Here's how the part is built. I have some questions about the finished solid (model axes, mm). A direction names the side the tool comes from. Round coordinates to 2 decimals unless told otherwise and drop trailing zeros. Loops run counter-clockwise (first coordinate to the right, second up) from the corner with the lowest first, then second, coordinate; pieces in that order, holes last. Notation, with made-up numbers: M 31.25,-23 L 44.25,-23 A12 cw 44.25,-9 Z; hole C 43.25,-3 d1. An arc over 180 degrees is marked long. Answer as CSV lines item,"result".
```python
from build123d import *


with BuildPart() as part:
    # Sweep1: sweep along a path in Sketch2
    with BuildLine(Plane.XY) as sweep1_path:
        Line((0.760799283, -6.022132882), (48.345774261, -0.010539388))
        ThreePointArc((48.345774261, -0.010539388), (62.299537257, -12.415218786), (48.142681566, -24.587605966))
        Line((48.142681566, -24.587605966), (0.663551745, -17.790449832))
        ThreePointArc((0.663551745, -17.790449832), (0.04348261, -17.733939776), (-0.579113336, -17.741247775))
        Line((-0.579113336, -17.741247775), (-238.647292697, -32.77092096))
        ThreePointArc((-238.647292697, -32.77092096), (-262.989356674, -9.727192609), (-238.269798997, 12.91111482))
        Line((-238.269798997, 12.91111482), (-0.482509205, -6.050792086))
        ThreePointArc((-0.482509205, -6.050792086), (0.139880947, -6.068388033), (0.760799283, -6.022132882))
    # Sketch3 → Sweep1 (sweep)
    with BuildSketch(Plane(origin=(-238.269798997, 12.91111482, 0), x_dir=(0, 0, 1), z_dir=(-0.9968355989946425, 0.07949080812894212, 0))):
        Polygon((0, 0), (5, 0), (5, 1.14), (-5, 1.14), (-5, 0), align=None)
    sweep(path=sweep1_path.line)


solid = part.part
```
1. For P1, Ø1, axis at x = -99.5, z = -2.5, coming from the +Y side; P2, Ø3, axis at x = -226.5, z = 2.5, coming from the +Y side; P3, Ø1.5, axis at x = -57, z = -3.5, coming from the +Y side; P4, Ø1.5, axis at x = -108.5, y = 5, coming from the -Z side, each with a flat end and sliding along its axis, tell me the tip position at first contact or that it passes through.
Evaluation:
P1,"stops at y = 3.03"
P2,"stops at y = 13.24"
P3,"stops at y = -0.34"
P4,"passes through"
2. If I drill on line 1 (Y direction, x = -69.5, z = 3.75); line 2 (Y direction, x = -54, z = 4); line 3 (X direction, y = -8, z = -1.25), over which ranges is the centre line in solid material (lowest first)? Write a range as [from, to].
Evaluation:
line 1,"y = [-23.23, -22.09], [-0.55, 0.6]"
line 2,"y = [-22.26, -21.11], [-1.78, -0.64]"
line 3,"x = [-264.05, -262.91], [61.53, 62.73]"
3. Which directions (+Z, -Z, +X, -X, +Y, -Y) give clear straight access to the entire face, cutting with the end or side of a thin tool? Please do faces 1 (the flat face through (23.91, -22.27, 0.07)), 2 (the flat face through (24.743, -1.843, 0.07)), 3 (the flat face through (-121.28, -25.36, -0.07)), 4 (the flat face through (-74, -23, -5)).
Evaluation:
face 1,"+Z, -Z, -Y"
face 2,"+Z, -Z, +Y"
face 3,"+Z, -Z"
face 4,"-Z, +X, -X, +Y, -Y"
4. I want a section at C-C, the plane y = 8.5. Please give me the cut outline in (x, z), and give its area (3 significant figures).
Evaluation:
outline,"M -255.54,-5 L -253.7,-5 L -253.7,5 L -255.54,5 Z; M -182.95,-5 L -168.61,-5 L -168.61,5 L -182.95,5 Z"
area,"162 mm²"
5. I want a section at B-B, the plane x = 36. Please give me the cut outline in (y, z).
Evaluation:
outline,"M -24,-5 L -22.85,-5 L -22.85,5 L -24,5 Z; M -1.57,-5 L -0.42,-5 L -0.42,5 L -1.57,5 Z"
6. I want a section at A-A, the plane z = -1. Please give me the cut outline in (x, y).
Evaluation:
outline,"M -238.58,-33.91 L -0.51,-18.88 A4.93 cw 0.5,-18.92 L 47.98,-25.72 A13.54 ccw long 48.2,1.12 L 0.62,-4.89 A4.93 cw -0.39,-4.91 L -238.18,14.05 A24.04 ccw long Z; hole M -238.65,-32.77 L -0.58,-17.74 A6.07 cw 0.66,-17.79 L 48.14,-24.59 A12.4 ccw long 48.35,-0.01 L 0.76,-6.02 A6.07 cw -0.48,-6.05 L -238.27,12.91 A22.9 ccw long Z"
